Job drawing, mm, ordinate dimensions from the low corner. One solid piece. A direction names the side the tool comes from. Coordinates: 2 decimals unless noted, no trailing zeros. Loops run counter-clockwise (first coordinate to the right, second up) from the corner with the lowest first, then second, coordinate; pieces in that order, holes last. Notation, with made-up numbers: (80, -25) - (126, -25) arc R19 cw to (126, 4) - close; hole circle Ø1 at (29.25, 54). An arc over 180 degrees is marked (long way). Use a Markdown table: item, result. Add a question column.
1) Band-saw the part on B-B (z = 3.2). Give the cut face in (x, y).
2) Tool access for the marked faces 4 and 5: list every direction of +Z, -Z, +X, -X, +Y, -Y with a clear straight run to the whole face (end or side of a thin tool).
3) Drop a flat-ended pin along its axis: P1, Ø1, axis at y = 1, z = 3.5, coming from the -X side. Give the stop position or say it passes through.
4) Pull direction X, two halves, no side cores. Call the marked faces 1, 2 and 3: +X half, -X half, draft (parallel to the pull), parting line (faces both ways), or undercut.
5) Band-saw the part on A-A (x = 5). Give the cut face in (y, z), plus the area to 3 significant figures.
6) Probe probe 1 along Y at (x, z) = (5, 3.9); probe 2 along X at (y, z) = (5.75, 3.8); probe 3 along Y at (x, z) = (5, 0.25). List the from-to ranges inside material, lowest first. Write a range as [from, to].
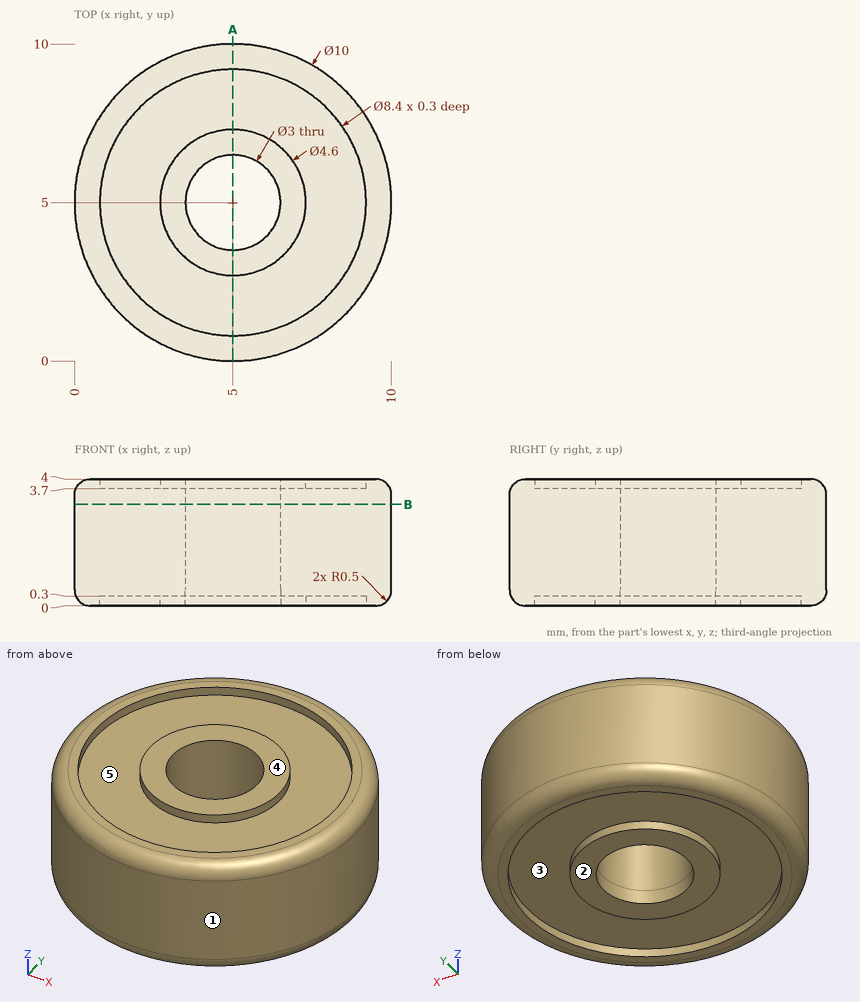
Answer block:
| question | item | result |
|---|---|---|
| 1 | outline | circle Ø10 at (5, 5); hole circle Ø3 at (5, 5) |
| 2 | face 4 | +Z, +X, -X, +Y, -Y |
| 2 | face 5 | +Z |
| 3 | P1 | x = 1.43 |
| 4 | face 1 | parting line |
| 4 | face 2 | draft |
| 4 | face 3 | undercut |
| 5 | outline | (0, 0.5) arc R0.5 ccw to (0.5, 0) - (0.8, 0) - (0.8, 0.3) - (2.7, 0.3) - (2.7, 0) - (3.5, 0) - (3.5, 4) - (2.7, 4) - (2.7, 3.7) - (0.8, 3.7) - (0.8, 4) - (0.5, 4) arc R0.5 ccw to (0, 3.5) - close; (6.5, 0) - (7.3, 0) - (7.3, 0.3) - (9.2, 0.3) - (9.2, 0) - (9.5, 0) arc R0.5 ccw to (10, 0.5) - (10, 3.5) arc R0.5 ccw to (9.5, 4) - (9.2, 4) - (9.2, 3.7) - (7.3, 3.7) - (7.3, 4) - (6.5, 4) - close |
| 5 | area | 25.5 mm2 |
| 6 | probe 1 | [0.2, 0.8], [2.7, 3.5], [6.5, 7.3], [9.2, 9.8] |
| 6 | probe 2 | [0.16, 0.87], [2.83, 3.7], [6.3, 7.17], [9.13, 9.84] |
| 6 | probe 3 | [0.07, 0.8], [2.7, 3.5], [6.5, 7.3], [9.2, 9.93] |
